```python
from build123d import *

# Parameters (mm, degrees)
SKETCH1_W               = 70
SKETCH1_H               = 349.15
SKETCH1_R               = 6.425
SKETCH1_R_2             = 2.5
SKETCH1_W_2             = 20.5
SKETCH1_H_2             = 40.7
BOSS_EXTRUDE1_DEPTH     = 3.1
CUT_EXTRUDE1_DEPTH      = 1
CUT_EXTRUDE1_DEPTH_BACK = 4.1
FILLET2_R               = 30
SKETCH4_R               = 3.25
SKETCH4_W               = 35
SKETCH4_H               = 3.1
CUT_EXTRUDE2_DEPTH      = 4.1


with BuildPart() as part:
    # Sketch1 → Boss-Extrude1 (new body)
    with BuildSketch(Plane.XY):
        Rectangle(SKETCH1_W, SKETCH1_H)
        with Locations((0, -139.575)):
            Circle(SKETCH1_R, mode=Mode.SUBTRACT)
        with Locations((-5, 74.575)):
            Circle(SKETCH1_R_2, mode=Mode.SUBTRACT)
        with Locations((5, 74.575)):
            Circle(SKETCH1_R_2, mode=Mode.SUBTRACT)
        with Locations((5, 25.575)):
            Circle(SKETCH1_R_2, mode=Mode.SUBTRACT)
        with Locations((-5, 25.575)):
            Circle(SKETCH1_R_2, mode=Mode.SUBTRACT)
        with Locations((0, 50.075)):
            Rectangle(SKETCH1_W_2, SKETCH1_H_2, mode=Mode.SUBTRACT)
    extrude(amount=BOSS_EXTRUDE1_DEPTH)

    # Sketch2 → Cut-Extrude1 (cut, two sides)
    with BuildSketch(Plane.XY.offset(3.1)) as cut_extrude1_sk:
        with BuildLine():
            Line((-16, -136.269781362), (-35, -74.575))
            Line((-35, -74.575), (-35, -174.575))
            Line((-35, -174.575), (35, -174.575))
            Line((35, -174.575), (35, -74.575))
            Line((35, -74.575), (16, -136.269781362))
            ThreePointArc((16, -136.269781362), (0, -150.051383336), (-16, -136.269781362))
        make_face()
    extrude(amount=CUT_EXTRUDE1_DEPTH, mode=Mode.SUBTRACT)
    extrude(cut_extrude1_sk.sketch, amount=-CUT_EXTRUDE1_DEPTH_BACK, mode=Mode.SUBTRACT)

    # Fillet2
    fillet2_edges = [part.edges().sort_by_distance(p)[0] for p in [
        (-35, -74.575, 1.55),
        (35, -74.575, 1.55),
    ]]
    fillet(fillet2_edges, radius=FILLET2_R)

    # Sketch4 → Cut-Extrude2 (cut, through all)
    with BuildSketch(Plane.XY.offset(3.1)):
        with Locations((0, 122.675)):
            Circle(SKETCH4_R)
        with Locations((0, 151.475)):
            Circle(SKETCH4_R)
        with Locations((-17.5, 173.025)):
            Rectangle(SKETCH4_W, SKETCH4_H)
        with Locations((-17.5, 101.125)):
            Rectangle(SKETCH4_W, SKETCH4_H)
    extrude(amount=-CUT_EXTRUDE2_DEPTH, mode=Mode.SUBTRACT)


solid = part.part
```
The listing builds one solid part. Answer for the finished solid, in the listing's coordinates (mm). Coordinates: 2 decimals unless noted, no trailing zeros. Loops run counter-clockwise (first coordinate to the right, second up) from the corner with the lowest first, then second, coordinate; pieces in that order, holes last. Notation, with made-up numbers: M 70.25,39 L 84.25,39 A16 ccw 84.25,62 Z; hole C 36.25,54.5 d8. An arc over 180 degrees is marked long. Answer as CSV lines item,"result". Start each with the question number.
(1) Find the intervals of material crossed by L1, parallel to X at y = 37.5, z = 0.45; L2, parallel to X at y = 74, z = 2.8; L3, parallel to Y at x = -5, z = 1.95 (3 decimals), in increasing order. Write a range as [from, to].
(2) The mould has two halves that part along X. Classify faces 1 (the cylindrical face through (0.32, -150.05, 1.57)), 2 (the cylindrical face through (-0.7, 148.3, 1.6)), 3 (the flat face through (-24.712, -107.982, 1.572)): pulls with the +X half, pulls with the -X half, needs draft (parallel to the pull), parting line crosses it, or undercut.
(3) The part is cut by section C-C (z = 1.1). State how many separate pieces and enclosed holes the cut face has, and give its area (3 significant figures).
(4) The part is cut by section A-A (y = 58.5). Give the vertices of the cut face in (x, z).
(5) Given pin 1 (4.5 mm diameter, centred on x = 5, y = 25.575, fed in from -Z); pin 2 (1.6 mm diameter, centred on y = 173, z = 1.5, fed in from -X); pin 3 (1.6 mm diameter, centred on x = -18.5, z = 1, fed in from +Y) (3 decimals), each flat-ended and moving along its own axis, determine where each tip first touches the part or whether it passes through.
(6) The part is cut by section D-D (y = -129.5). Give the vertices of the cut face in (x, z).
(7) The part is cut by section B-B (x = -24.5). Give the vertices of the cut face in (y, z) (3 decimals), and give its area (3 significant figures).
Determined:
1,L1,"[-35, -10.25], [10.25, 35]"
1,L2,"[-35, -7.43], [-2.57, 2.57], [7.43, 35]"
1,L3,"[-149.259, -143.61], [-135.54, 23.075], [28.075, 29.725], [70.425, 72.075], [77.075, 99.575], [102.675, 171.475]"
2,face 1,"parting line crosses it"
2,face 2,"undercut"
2,face 3,"pulls with the -X half"
3,separate pieces,"1"
3,enclosed holes,"8"
3,area,"19,600 mm2"
4,outline,"M -35,0 L -10.25,0 L -10.25,3.1 L -35,3.1 Z; M 10.25,0 L 35,0 L 35,3.1 L 10.25,3.1 Z"
5,pin 1,"through"
5,pin 2,"x = 0"
5,pin 3,"y = 171.475"
6,outline,"M -18.08,0 L 18.08,0 L 18.08,3.1 L -18.08,3.1 Z"
7,outline,"M -108.669,0 L 99.575,0 L 99.575,3.1 L -108.669,3.1 Z; M 102.675,0 L 171.475,0 L 171.475,3.1 L 102.675,3.1 Z"
7,area,"859 mm2"
